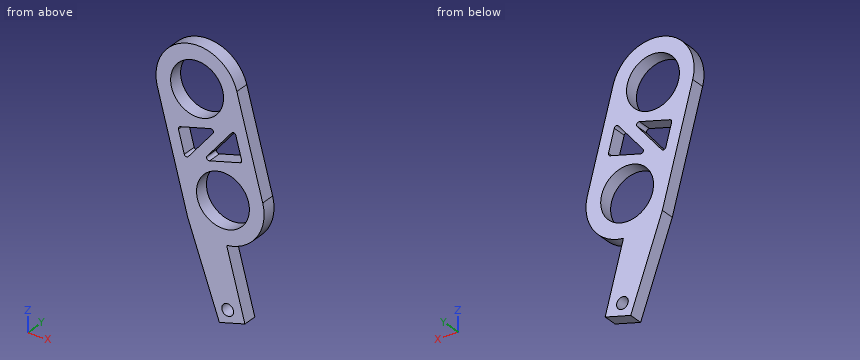
```python
from build123d import *

# Parameters (mm, degrees)
SKETCH1_R           = 14.2875
BOSS_EXTRUDE1_DEPTH = 7.62
CUT_EXTRUDE1_DEPTH  = 8.62
FILLET1_R           = 1.27
SKETCH3_R           = 3.175
CUT_EXTRUDE2_DEPTH  = 7.62


with BuildPart() as part:
    # Sketch1 → Boss-Extrude1 (new body)
    with BuildSketch(Plane(origin=(0, 0, 0), x_dir=(1, 0, 0), z_dir=(0, 1, 0))):
        with BuildLine():
            Line((7.49794353, -57.888099751), (21.467701489, -5.752253277))
            ThreePointArc((21.467701489, -5.752253277), (18.22000551, 12.727215887), (1.986922694, 22.136006036))
            Line((1.986922694, 22.136006036), (11.847928312, 58.937780017))
            Line((11.847928312, 58.937780017), (-1.952736931, 62.635657124))
            Line((-1.952736931, 62.635657124), (-19.044132712, 14.797135091))
            Line((-19.044132712, 14.797135091), (-35.437459449, -46.383593197))
            ThreePointArc((-35.437459449, -46.383593197), (-19.722011237, -73.603547963), (7.49794353, -57.888099751))
        make_face()
        with Locations((-13.969757959, -52.135846474)):
            Circle(SKETCH1_R, mode=Mode.SUBTRACT)
        Circle(SKETCH1_R, mode=Mode.SUBTRACT)
    extrude(amount=BOSS_EXTRUDE1_DEPTH)

    # Sketch2 → Cut-Extrude1 (cut, through all)
    with BuildSketch(Plane(origin=(0, 7.62, 0), x_dir=(1, 0, 0), z_dir=(0, 1, 0))):
        Polygon((-20.265778136, -14.291812351), (-2.906828988, -35.378138121), (-24.374530477, -29.625884844), align=None)
        Polygon((-11.064131806, -16.757386054), (10.403569683, -22.509639332), (6.294817342, -37.843711824), align=None)
    extrude(amount=-CUT_EXTRUDE1_DEPTH, mode=Mode.SUBTRACT)

    # Fillet1
    fillet1_edges = [part.edges().sort_by_distance(p)[0] for p in [
        (-24.374530477, 3.81, 29.625884844),
        (-20.265778136, 3.81, 14.291812351),
        (-2.906828988, 3.81, 35.378138121),
        (6.294817342, 3.81, 37.843711824),
        (-11.064131806, 3.81, 16.757386054),
        (10.403569683, 3.81, 22.509639332),
    ]]
    fillet(fillet1_edges, radius=FILLET1_R)

    # Sketch3 → Cut-Extrude2 (cut)
    with BuildSketch(Plane(origin=(0, 7.62, 0), x_dir=(1, 0, 0), z_dir=(0, 1, 0))):
        with Locations((2.537391129, 54.858527191)):
            Circle(SKETCH3_R)
    extrude(amount=-CUT_EXTRUDE2_DEPTH, mode=Mode.SUBTRACT)


solid = part.part
```
The listing builds one solid part. Answer for the finished solid, in the listing's coordinates (mm). Round coordinates to 2 decimals unless told otherwise and drop trailing zeros. Loops run counter-clockwise (first coordinate to the right, second up) from the corner with the lowest first, then second, coordinate; pieces in that order, holes last.
Q1. Section B-B, the plane z = 26 is taken. Determine the outline of the cut face in (x, y).
Q2. Given pin 1 Ø17 at (x, z) = (0, 0) entering from +Y, flat-ended and moving along its own axis, determine where the tip first touches the part or whether it passes through.
Q3. Section D-D, the plane y = 2.75 is taken. Count the separate pieces of the cut face and the enclosed holes in it, then the cut area to 3 significant figures.
Q4. Section A-A, the plane x = 3.5 is taken. Determine the outline of the cut face in (y, z).
Q5. Section C-C, the plane z = 65 is taken. Determine the outline of the cut face in (x, y).
Q6. Find the intervals of material crossed by line 1 (X direction, y = 6, z = 28); line 2 (X direction, y = 0.5, z = 47); line 3 (X direction, y = 7.25, z = 51.5), in increasing order.
Completed:
1. outline: (-29.98, 0) - (-23.4, 0) - (-23.4, 7.62) - (-29.98, 7.62) - close; (-10.63, 0) - (-3.46, 0) - (-3.46, 7.62) - (-10.63, 7.62) - close; (9.47, 0) - (16.04, 0) - (16.04, 7.62) - (9.47, 7.62) - close
2. pin 1: passes through
3. separate pieces: 1
3. enclosed holes: 5
3. area: 2,990 mm2
4. outline: (0, -61.17) - (7.62, -61.17) - (7.62, -57.88) - (0, -57.88) - close; (0, -51.83) - (7.62, -51.83) - (7.62, -27.78) - (0, -27.78) - close; (0, -21.95) - (7.62, -21.95) - (7.62, -13.85) - (0, -13.85) - close; (0, 13.85) - (7.62, 13.85) - (7.62, 20.66) - (0, 20.66) - close; (0, 34.45) - (7.62, 34.45) - (7.62, 65.87) - (0, 65.87) - close
5. outline: (-32.09, 0) - (-20.19, 0) - (-20.19, 7.62) - (-32.09, 7.62) - close; (-7.75, 0) - (4.15, 0) - (4.15, 7.62) - (-7.75, 7.62) - close
6. line 1: x = -30.51 to -23.94, -8.98 to -1.81, 8.93 to 15.51
6. line 2: x = -35.59 to -27.3, -0.64 to 10.42
6. line 3: x = -36.19 to -28.24, 0.3 to 9.21
